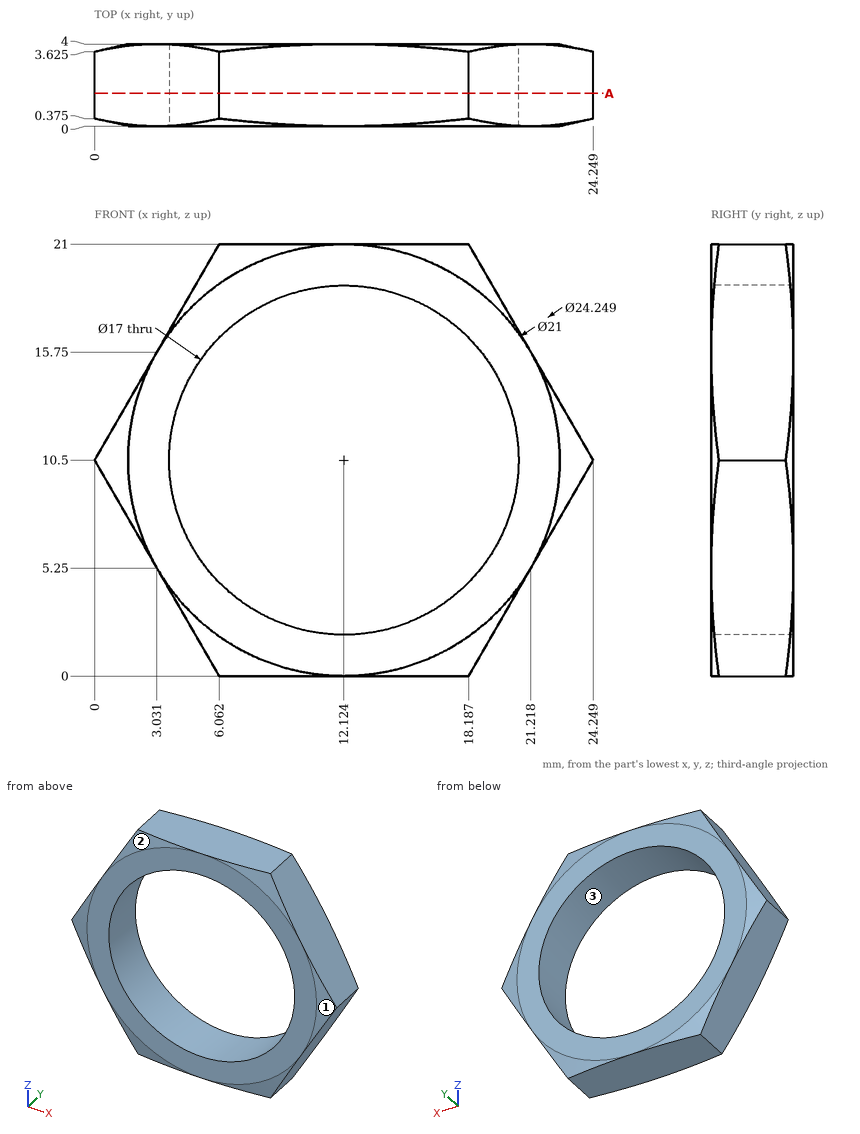
Geometry: see drawing. Coordinates: mm, zero at the bounding-box minimum. Coordinates: 2 decimals unless noted, no trailing zeros. Order: outer loops, then holes, each group sorted by start corner. A loop starts at its lowest first (then second) coordinate and runs counter-clockwise, first axis right, second up. Notation, with made-up numbers: M -39.5,-14 L -17.5,-14 A27 cw -17.5,20 Z; hole C 70,1 d11. An arc over 180 degrees is marked long. Write item = value, one per line. Start each with the question number.
(1) First-contact query: P1, Ø1, axis at y = 0.5, z = 9, coming from the -X side; P2, Ø10, axis at x = 12.12, z = 10.5, coming from the -Y side. Flat tips, straight axial feed; report the tip coordinate or a pass-through.
(2) Line query: line 1 along Z through (x, y) = (12, 3.1); line 2 along X through (y, z) = (1.3, 7.5) (1 decimal); line 3 along Z through (x, y) = (14, 3.4). Output: solid intervals per line, ascending. Write a range as [from, to].
(3) Pull-direction query (X, two-part tool) for the marked faces 1, 2 and 3; classes: released by +X, released by -X, zero draft, split by the parting line, or undercut.
(4) Section A-A on y = 1.6. Output: boundary loops of the cut face in (x, z) (1 decimal), and give its area (3 significant figures).
Result set:
q1.P1 = 0.58
q1.P2 = through
q2.line_1 = [0, 2], [19, 21]
q2.line_2 = [1.7, 4.2], [20.1, 22.5]
q2.line_3 = [0, 2.21], [18.79, 21]
q3.face_1 = released by +X
q3.face_2 = released by -X
q3.face_3 = undercut
q4.outline = M 0,10.5 L 6.1,0 L 18.2,0 L 24.2,10.5 L 18.2,21 L 6.1,21 Z; hole C 12.1,10.5 d17
q4.area = 155 mm²
